The listing builds one solid part. Answer for the finished solid, in the listing's coordinates (mm). Round coordinates to 2 decimals unless told otherwise and drop trailing zeros. Write each loop counter-clockwise with the first axis right and the second up, starting at its lowest first coordinate (ties: lowest second). Pieces come first, ordered by that corner, then holes.
(1) Each of these flat-tipped pins is pushed along its axis until it touches: pin 1 Ø2 at (y, z) = (120.5, -1) entering from -X; pin 2 Ø3 at (x, z) = (9.5, -29) entering from +Y; pin 3 Ø3 at (x, y) = (-14, 169) entering from +Z; pin 4 Ø14.5 at (y, z) = (101.6, -68.1) entering from +X. Where does it stop, or does it pass through?
(2) Find the intervals of material crossed by probe 1 along X at (y, z) = (107.5, 0.5); probe 2 along X at (y, z) = (91, 13.5); probe 3 along Y at (x, z) = (2.25, -68.1), in increasing order.
(3) A cutting plane is placed at B-B, the plane x = 15. Give the vertices of the cut face in (y, z).
(4) A cutting plane is placed at A-A, the plane z = 0. Give the vertices of the cut face in (x, y), and give its area (3 significant figures).
(5) A cutting plane is placed at C-C, the plane y = 72. Give the vertices of the cut face in (x, z), and give its area (3 significant figures).
(6) The mould has two halves that part along X. Classify faces 1 (the face through (-12.7, 101, -47)), 2 (the face through (12.7, 101, -47)), 3 (the face through (-15.456, 100.178, -20.157)), 4 (the face through (0.178, 81.713, -51.638)): +X half, -X half, draft (parallel to the pull), parting line (faces both ways), or undercut.
(7) A cutting plane is placed at D-D, the plane y = 159. Give the vertices of the cut face in (x, z), and give its area (3 significant figures).
from build123d import *

# Parameters (mm, degrees)
SKETCH1_R                            = 30
SKETCH1_R_2                          = 25.4
BOSS_EXTRUDE1_DEPTH                  = 203.2
SKETCH2_W                            = 25.4
SKETCH2_H                            = 63.5
BOSS_EXTRUDE2_DEPTH                  = 50.8
BOSS_EXTRUDE2_DIRECTION_2_REACH      = 215.987
BOSS_EXTRUDE2_DIRECTION_2_END_RADIUS = 30
CUT_EXTRUDE3_REACH                   = 224.805
SKETCH3_R                            = 6.35
CUT_EXTRUDE3_DIRECTION_2_DEPTH       = 223.805228843


with BuildPart() as part:
    # Sketch1 → Boss-Extrude1 (new body)
    with BuildSketch(Plane(origin=(0, 0, 0), x_dir=(1, 0, 0), z_dir=(0, 1, 0))):
        with Locations(Location((0, 0, 0), (0, 0, 270))):
            Circle(SKETCH1_R)
        with Locations(Location((0, 0, 0), (0, 0, 270))):
            Circle(SKETCH1_R_2, mode=Mode.SUBTRACT)
    extrude(amount=BOSS_EXTRUDE1_DEPTH)

    # Sketch2 → Boss-Extrude2 (add)
    with BuildSketch(Plane(origin=(0, 0, -30), x_dir=(-1, 0, 0), z_dir=(0, 0, -1))):
        with Locations((0, 101.6)):
            Rectangle(SKETCH2_W, SKETCH2_H)
    extrude(amount=BOSS_EXTRUDE2_DEPTH)

    # Boss-Extrude2 direction 2: up to this cylinder (the profile starts outside it)
    boss_extrude2_direction_2_end = Plane(origin=(0, 101.6, 0), z_dir=(0, -1, 0)) * Cylinder(BOSS_EXTRUDE2_DIRECTION_2_END_RADIUS, 492.974, mode=Mode.PRIVATE)
    # Sketch2 → Boss-Extrude2 direction 2 (add, up to the surface)
    with BuildSketch(Plane(origin=(0, 0, -30), x_dir=(-1, 0, 0), z_dir=(0, 0, -1)), mode=Mode.PRIVATE) as boss_extrude2_direction_2_sk1:
        with Locations((0, 101.6)):
            Rectangle(SKETCH2_W, SKETCH2_H)
    boss_extrude2_direction_2_tool1 = extrude(boss_extrude2_direction_2_sk1.sketch, amount=-BOSS_EXTRUDE2_DIRECTION_2_REACH, mode=Mode.PRIVATE) - boss_extrude2_direction_2_end
    add(boss_extrude2_direction_2_tool1.solids().sort_by_distance((0, 101.6, -30))[0])
    add(boss_extrude2_direction_2_tool1.solids().sort_by_distance((0, 101.6, -30))[1])

    # Sketch3 → Cut-Extrude3 (cut, up to next)
    with BuildSketch(Plane(origin=(12.7, 0, 0), x_dir=(0, 0, -1), z_dir=(1, 0, 0)), mode=Mode.PRIVATE) as cut_extrude3_sk1:
        with BuildLine():
            Line((72.678913322, 93.247804014), (30, 69.85))
            Line((30, 69.85), (80.8, 69.85))
            Line((80.8, 69.85), (80.8, 133.35))
            Line((80.8, 133.35), (30, 133.35))
            Line((30, 133.35), (72.678913322, 109.952195986))
            ThreePointArc((72.678913322, 109.952195986), (76.295723714, 106.453425368), (77.625, 101.6))
            ThreePointArc((77.625, 101.6), (76.295723714, 96.746574632), (72.678913322, 93.247804014))
        make_face()
    cut_extrude3_tool1 = extrude(cut_extrude3_sk1.sketch, amount=-CUT_EXTRUDE3_REACH, mode=Mode.PRIVATE) & part.part
    # Sketch3 → Cut-Extrude3 (cut, up to next)
    with BuildSketch(Plane(origin=(12.7, 0, 0), x_dir=(0, 0, -1), z_dir=(1, 0, 0)), mode=Mode.PRIVATE) as cut_extrude3_sk2:
        with Locations(Location((68.1, 101.6, 0), (0, 0, 270))):
            Circle(SKETCH3_R)
    cut_extrude3_tool2 = extrude(cut_extrude3_sk2.sketch, amount=-CUT_EXTRUDE3_REACH, mode=Mode.PRIVATE) & part.part
    add(cut_extrude3_tool1.solids().sort_by_distance((12.7, 80.835833, -51.730381))[0], mode=Mode.SUBTRACT)
    add(cut_extrude3_tool2.solids().sort_by_distance((12.7, 101.6, -68.1))[0], mode=Mode.SUBTRACT)

    # Sketch3 → Cut-Extrude3 direction 2 (cut)
    with BuildSketch(Plane(origin=(12.7, 0, 0), x_dir=(0, 0, -1), z_dir=(1, 0, 0))):
        with BuildLine():
            Line((72.678913322, 93.247804014), (30, 69.85))
            Line((30, 69.85), (80.8, 69.85))
            Line((80.8, 69.85), (80.8, 133.35))
            Line((80.8, 133.35), (30, 133.35))
            Line((30, 133.35), (72.678913322, 109.952195986))
            ThreePointArc((72.678913322, 109.952195986), (76.295723714, 106.453425368), (77.625, 101.6))
            ThreePointArc((77.625, 101.6), (76.295723714, 96.746574632), (72.678913322, 93.247804014))
        make_face()
        with Locations(Location((68.1, 101.6, 0), (0, 0, 270))):
            Circle(SKETCH3_R)
    extrude(amount=CUT_EXTRUDE3_DIRECTION_2_DEPTH, mode=Mode.SUBTRACT)


solid = part.part
Solutions:
1. pin 1: stops at x = -30
1. pin 2: stops at y = 203.2
1. pin 3: stops at z = 27.27
1. pin 4: stops at x = 12.7
2. probe 1: x = -30 to -25.4, 25.4 to 30
2. probe 2: x = -26.79 to -21.52, 21.52 to 26.79
2. probe 3: y = 90.74 to 95.25, 107.95 to 112.46
3. outline: (0, -25.98) - (203.2, -25.98) - (203.2, -20.5) - (0, -20.5) - close; (0, 20.5) - (203.2, 20.5) - (203.2, 25.98) - (0, 25.98) - close
4. outline: (-30, 0) - (-25.4, 0) - (-25.4, 203.2) - (-30, 203.2) - close; (25.4, 0) - (30, 0) - (30, 203.2) - (25.4, 203.2) - close
4. area: 1,870 mm2
5. outline: (-12.7, -33.92) - (12.7, -33.92) - (12.7, -27.18) arc R30 ccw (long way) to (-12.7, -27.18) - close; hole circle Ø50.8 at (0, 0)
5. area: 924 mm2
6. face 1: -X half
6. face 2: +X half
6. face 3: undercut
6. face 4: draft
7. outline: circle Ø60 at (0, 0); hole circle Ø50.8 at (0, 0)
7. area: 801 mm2
